Here's how the part is built. I have some questions about the finished solid (model axes, mm). Face numbers are marked on the shaded views. A direction names the side the tool comes from. Give positions to 0.01 mm unless a question says otherwise; leave off trailing zeros. Loops run counter-clockwise (first coordinate to the right, second up) from the corner with the lowest first, then second, coordinate; pieces in that order, holes last. Notation, with made-up numbers: (-15, 78) -> (39, 78) arc R20 cw to (39, 83) -> close; hole circle Ø7 at (82, -7.75). An arc over 180 degrees is marked (long way). Answer in a Markdown table with one row per item. Add a question column.
Item 1: Which directions (+Z, -Z, +X, -X, +Y, -Y) give clear straight access to the entire face, cutting with the end or side of a thin tool? Please do the marked faces 1, 2 and 3.
Item 2: If I drill on line 1 (X direction, y = 12.7, z = 10); line 2 (Y direction, x = -38.1, z = 10); line 3 (Z direction, x = -28, y = 14), over which ranges is the centre line in solid material (lowest first)?
Item 3: If we section it at C-C (y = 17.75): Write out the boundary of the cut face in (x, z).
Item 4: For P1, Ø3, axis at y = 22, z = 23, coming from the +X side; P2, Ø4, axis at y = 4, z = 27.5, coming from the -X side; P3, Ø2, axis at x = -60, y = 8, coming from the +Z side; P4, Ø12, axis at y = 3, z = 28, coming from the +X side, each with a flat end and sliding along its axis, tell me the tip position at first contact or that it passes through.
Item 5: If we section it at B-B (x = -38.1): Write out the boundary of the cut face in (y, z), then the cut area to 3 significant figures.
Item 6: If we section it at A-A (z = 28): Write out the boundary of the cut face in (x, y).
Item 7: If we section it at D-D (z = 5): Write out the boundary of the cut face in (x, y).
Item 8: We'd pull the mould along X, two halves only. Please class the marked faces 4, 5 and 6: released by +X, released by -X, zero draft, split by the parting line, or undercut.
```python
from build123d import *

# Parameters (mm, degrees)
F0_W     = 76.2
F0_H     = 25.4
F1_DEPTH = 19.05
F2_W     = 12.7
F2_H     = 12.7
F3_DEPTH = 12.7
F4_R     = 6.35
F5_DEPTH = 19.05


with BuildPart() as f1:
    # F0 (on Top) → F1 (new body)
    with BuildSketch(Plane.XY):
        with Locations((-38.1, 12.7)):
            Rectangle(F0_W, F0_H)
    extrude(amount=F1_DEPTH)

    # F2 (on face) → F3 (join)
    with BuildSketch(Plane.XY.offset(19.05)):
        with Locations((-69.85, 19.05)):
            Rectangle(F2_W, F2_H)
        with Locations((-6.35, 6.35)):
            Rectangle(F2_W, F2_H)
    extrude(amount=F3_DEPTH)

    # F4 (on face) → F5 (cut)
    with BuildSketch(Plane(origin=(0, 0, 0), x_dir=(1, 0, 0), z_dir=(0, 0, -1))):
        with Locations((-38.1, -12.7)):
            Circle(F4_R)
    extrude(amount=-F5_DEPTH, mode=Mode.SUBTRACT)


solid = f1.part
```
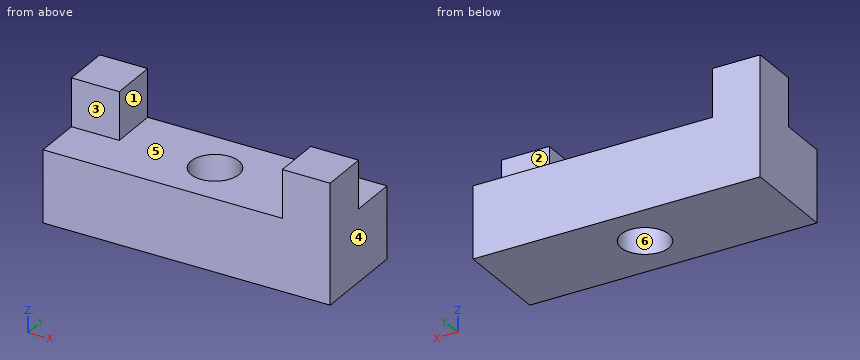
Recorded:
| question | item | result |
|---|---|---|
| 1 | face 1 | +Z, +X, +Y, -Y |
| 1 | face 2 | +Z, +X, +Y |
| 1 | face 3 | +Z, -X, -Y |
| 2 | line 1 | x = -76.2 to -44.45, -31.75 to 0 |
| 2 | line 2 | y = 0 to 6.35, 19.05 to 25.4 |
| 2 | line 3 | z = 0 to 19.05 |
| 3 | outline | (-76.2, 0) -> (-41.95, 0) -> (-41.95, 19.05) -> (-63.5, 19.05) -> (-63.5, 31.75) -> (-76.2, 31.75) -> close; (-34.25, 0) -> (0, 0) -> (0, 19.05) -> (-34.25, 19.05) -> close |
| 4 | P1 | stops at x = -63.5 |
| 4 | P2 | stops at x = -12.7 |
| 4 | P3 | stops at z = 19.05 |
| 4 | P4 | stops at x = 0 |
| 5 | outline | (0, 0) -> (6.35, 0) -> (6.35, 19.05) -> (0, 19.05) -> close; (19.05, 0) -> (25.4, 0) -> (25.4, 19.05) -> (19.05, 19.05) -> close |
| 5 | area | 242 mm^2 |
| 6 | outline | (-76.2, 12.7) -> (-63.5, 12.7) -> (-63.5, 25.4) -> (-76.2, 25.4) -> close; (-12.7, 0) -> (0, 0) -> (0, 12.7) -> (-12.7, 12.7) -> close |
| 7 | outline | (-76.2, 0) -> (0, 0) -> (0, 25.4) -> (-76.2, 25.4) -> close; hole circle Ø12.7 at (-38.1, 12.7) |
| 8 | face 4 | released by +X |
| 8 | face 5 | zero draft |
| 8 | face 6 | undercut |
